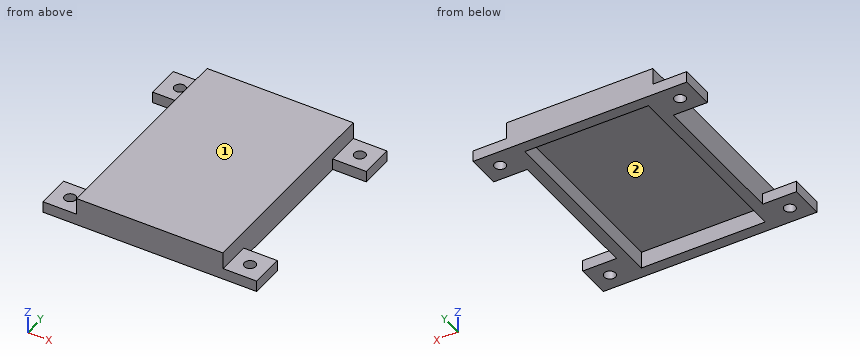
from build123d import *

# Parameters (mm, degrees)
SKETCH_1_W          = 26
SKETCH_1_H          = 38
EXTRUDE_1_DEPTH     = 5
SKETCH_2_W          = 22
SKETCH_2_H          = 34
CUT_EXTRUDE_1_DEPTH = 3
SKETCH_4_W          = 6
SKETCH_4_H          = 6
EXTRUDE_2_DEPTH     = 2
SKETCH_5_R          = 1
CUT_EXTRUDE_4_DEPTH = 2


with BuildPart() as part:
    # ｽｹｯﾁ1 → ﾎﾞｽ - 押し出し1 (new body)
    with BuildSketch(Plane.XY):
        Rectangle(SKETCH_1_W, SKETCH_1_H)
    extrude(amount=EXTRUDE_1_DEPTH)

    # ｽｹｯﾁ2 → ｶｯﾄ - 押し出し1 (cut)
    with BuildSketch(Plane.XY):
        Rectangle(SKETCH_2_W, SKETCH_2_H)
    extrude(amount=CUT_EXTRUDE_1_DEPTH, mode=Mode.SUBTRACT)

    # ｽｹｯﾁ4 → ﾎﾞｽ - 押し出し2 (add)
    with BuildSketch(Plane.XY):
        with Locations((16, 16)):
            Rectangle(SKETCH_4_W, SKETCH_4_H)
        with Locations((16, -16)):
            Rectangle(SKETCH_4_W, SKETCH_4_H)
        with Locations((-16, -16)):
            Rectangle(SKETCH_4_W, SKETCH_4_H)
        with Locations((-16, 16)):
            Rectangle(SKETCH_4_W, SKETCH_4_H)
    extrude(amount=EXTRUDE_2_DEPTH)

    # ｽｹｯﾁ5 → ｶｯﾄ - 押し出し4 (cut)
    with BuildSketch(Plane.XY):
        with Locations((-16, 16)):
            Circle(SKETCH_5_R)
        with Locations((-16, -16)):
            Circle(SKETCH_5_R)
        with Locations((16, -16)):
            Circle(SKETCH_5_R)
        with Locations((16, 16)):
            Circle(SKETCH_5_R)
    extrude(amount=CUT_EXTRUDE_4_DEPTH, mode=Mode.SUBTRACT)


solid = part.part
Check sheet for the modelled part. Datum: model origin and axes. Units: mm. Face numbers are marked on the shaded views. Coordinates: 2 decimals unless noted, no trailing zeros. Write each loop counter-clockwise with the first axis right and the second up, starting at its lowest first coordinate (ties: lowest second). Pieces come first, ordered by that corner, then holes.
Item 1: Cross-section at A-A on z = 0.65. Record the boundary of the cut face in (x, y).
Numbers:
outline: (-19, -19) - (19, -19) - (19, -13) - (13, -13) - (13, 13) - (19, 13) - (19, 19) - (-19, 19) - (-19, 13) - (-13, 13) - (-13, -13) - (-19, -13) - close; hole circle Ø2 at (-16, -16); hole circle Ø2 at (-16, 16); hole (-11, -17) - (11, -17) - (11, 17) - (-11, 17) - close; hole circle Ø2 at (16, -16); hole circle Ø2 at (16, 16)
Item 2: Scan lines: probe 1 along Y at (x, z) = (16, 1.1); probe 2 along X at (y, z) = (-7, 0.6); probe 3 along Y at (x, z) = (6.5, 0.85). Record each from-to range of solid material in increasing order.
Numbers:
probe 1: y = -19 to -17, -15 to -13, 13 to 15, 17 to 19
probe 2: x = -13 to -11, 11 to 13
probe 3: y = -19 to -17, 17 to 19
Item 3: Depth check by flat-ended pin: pin 1 Ø1.5 at (y, z) = (-2.5, 2) entering from +X; pin 2 Ø2.5 at (y, z) = (-7.5, 1.5) entering from -X; pin 3 Ø3 at (x, y) = (-17.5, -15) entering from +Z. Enter the tip coordinate at first touch or a pass-through.
Numbers:
pin 1: stops at x = 13
pin 2: stops at x = -13
pin 3: stops at z = 2
Item 4: Cross-section at C-C on x = 16. Record the boundary of the cut face in (y, z), then the cut area to 3 significant figures.
Numbers:
outline: (-19, 0) - (-17, 0) - (-17, 2) - (-19, 2) - close; (-15, 0) - (-13, 0) - (-13, 2) - (-15, 2) - close; (13, 0) - (15, 0) - (15, 2) - (13, 2) - close; (17, 0) - (19, 0) - (19, 2) - (17, 2) - close
area: 16.0 mm2
Item 5: Cross-section at B-B on y = 16. Record the boundary of the cut face in (x, z), then the cut area to 3 significant figures.
Numbers:
outline: (-19, 0) - (-17, 0) - (-17, 2) - (-19, 2) - close; (-15, 0) - (-11, 0) - (-11, 3) - (11, 3) - (11, 0) - (15, 0) - (15, 2) - (13, 2) - (13, 5) - (-13, 5) - (-13, 2) - (-15, 2) - close; (17, 0) - (19, 0) - (19, 2) - (17, 2) - close
area: 80.0 mm2
Item 6: Cross-section at D-D on y = -9. Record the boundary of the cut face in (x, z).
Numbers:
outline: (-13, 0) - (-11, 0) - (-11, 3) - (11, 3) - (11, 0) - (13, 0) - (13, 5) - (-13, 5) - close
Item 7: Mould release check, pull along X, two halves, no side actions. Record for the marked faces 1 and 2: released by +X, released by -X, zero draft, split by the parting line, or undercut.
Numbers:
face 1: zero draft
face 2: undercut
